```python
from build123d import *

# Parameters (mm, degrees)
F0_R     = 59.319188
F1_DEPTH = 25
F3_R     = 33.106016
F4_DEPTH = 116.983913
F5_R     = 10


with BuildPart() as f1:
    # F0 (on Top) → F1 (new body)
    with BuildSketch(Plane.XY):
        Circle(F0_R)
    extrude(amount=F1_DEPTH)

    # F3 (on offset) → F4 (cut)
    with BuildSketch(Plane.XY.offset(50)):
        Circle(F3_R)
    extrude(amount=-F4_DEPTH, mode=Mode.SUBTRACT)

    # F5
    f5_edges = [f1.edges().sort_by_distance(p)[0] for p in [
        (-59.319188, 0, 0),
        (-59.319188, 0, 25),
    ]]
    fillet(f5_edges, radius=F5_R)


solid = f1.part
```
Can you work these out from the model? Positions are in its coordinate system, mm. Round coordinates to 2 decimals unless told otherwise and drop trailing zeros. Loops run counter-clockwise (first coordinate to the right, second up) from the corner with the lowest first, then second, coordinate; pieces in that order, holes last.
Item 1: Suppose I cut it at C-C, the plane z = 4. Write out the boundary of the cut face in (x, y).
Item 2: Please list where these lines run through material, in increasing order: L1, parallel to Y at x = -20, z = 18.5; L2, parallel to Z at x = 33.5, y = 37; L3, parallel to Y at x = -3, z = 1.
Item 3: If we mould it in two halves opening along Y, with no side actions, what happens to faces 1 (the flat face through (32, -10, 0)), 2 (the cylindrical face through (31.58, 9.94, 12.67)), 3 (the cylindrical face through (-12.9, -57.9, 12.5))? For each: +Y half, -Y half, draft (parallel to the pull), parting line (faces both ways), or undercut.
Item 4: Will these pins go through, and if not, where does the flat tip stop? pin 1 Ø3 at (y, z) = (18.5, 4) entering from -X; pin 2 Ø10 at (y, z) = (5.5, 11.5) entering from +X; pin 3 Ø8 at (x, z) = (47, 22) entering from +Y.
Item 5: Suppose I cut it at D-D, the plane z = 12. Write out the boundary of the cut face in (x, y).
Item 6: Suppose I cut it at A-A, the plane y = 0. Write out the boundary of the cut face in (x, z).
Reported:
1. outline: circle Ø114.64 at (0, 0); hole circle Ø66.21 at (0, 0)
2. L1: y = -55.17 to -26.38, 26.38 to 55.17
2. L2: z = 0.02 to 24.98
2. L3: y = -53.59 to -32.97, 32.97 to 53.59
3. face 1: draft
3. face 2: undercut
3. face 3: parting line
4. pin 1: stops at x = -55.37
4. pin 2: stops at x = 59.32
4. pin 3: stops at y = 38.33
5. outline: circle Ø118.64 at (0, 0); hole circle Ø66.21 at (0, 0)
6. outline: (-59.32, 10) arc R10 ccw to (-49.32, 0) - (-33.11, 0) - (-33.11, 25) - (-49.32, 25) arc R10 ccw to (-59.32, 15) - close; (33.11, 0) - (49.32, 0) arc R10 ccw to (59.32, 10) - (59.32, 15) arc R10 ccw to (49.32, 25) - (33.11, 25) - close
